Part model, mm, in its own coordinate system. A direction names the side the tool comes from. Round coordinates to 2 decimals unless told otherwise and drop trailing zeros. Write each question's results on one line, items separated by ' | '. Start each with the question number.
1. Drop flat-ended pins along their axis: pin 1 Ø3 at (x, z) = (-3, 5.5) entering from +Y; pin 2 Ø1 at (x, y) = (6.5, 12.5) entering from +Z; pin 3 Ø0.6 at (x, z) = (1, -5.5) entering from +Y. Give the stop position or say it passes through.
2. Which spindle directions (+Z, -Z, +X, -X, +Y, -Y) get a long thin tool onto all of the face, cutting with end or side? Do faces 4 (the face through (0, 4, -3)), 5 (the face through (0.1, 3.5, 0)), 6 (the face through (8.699, 0.285, 3.118)). Say none if no direction does.
3. Two-plate mould, pull along Z, no slides. Class faces 1 (the face through (0, 3, -2)), 2 (the face through (0.126, 4.285, -6.214)), 3 (the face through (0, 0, 4)): +Z half, -Z half, draft (parallel to the pull), parting line (faces both ways), or undercut.
4. Probe L1, parallel to Z at x = -4.75, y = 1; L2, parallel to Y at x = -6, z = -2.5; L3, parallel to Y at x = 5, z = -0.75. List the from-to ranges inside material, lowest first. Write a range as [from, to].
```python
from build123d import *

# Parameters (mm, degrees)
F1_DEPTH = 15
F4_DEPTH = 19
F5_R     = 1


with BuildPart() as f1:
    # F0 (on Front) → F1 (new body)
    with BuildSketch(Plane.XZ):
        Polygon((-9, 12.5), (-9, 0), (-9, -6.5152065011), (8.9999935767, -6.5152065011), (8.9999935767, 12.4847934989), align=None)
    extrude(amount=-F1_DEPTH)

    # F3 (on offset) → F4 (cut)
    with BuildSketch(Plane.YZ.offset(8.9999935767)):
        Polygon((3, -6.568428129), (3, -6.9065713324), (4, -6.9065713324), (4, 0), (3, 0), (3, -4.7258920968), (3.2896485645, -5.2308174782), (3.2896485645, -6.3381111249), align=None)
        with BuildLine():
            add(Edge.make_bspline(
                [(4, -6.9065713324), (7.8309681267, -7.469817996), (4.7241249122, 9.7180437297), (15.3055908158, 9.7582889721)],
                knots=[0, 0, 0, 0, 20.1378735884, 20.1378735884, 20.1378735884, 20.1378735884], degree=3))
            Line((4, -6.9065713324), (4, -7.8707002103))
            Line((4, -7.8707002103), (15.5558949336, -7.8707002103))
            Line((15.5558949336, -7.8707002103), (15.5558949336, -0.2191853659))
            Line((15.5558949336, -0.2191853659), (15.5479665846, 0.0968497843))
            Line((15.5479665846, 0.0968497843), (15.3055908158, 9.7582889721))
        make_face()
    extrude(amount=-F4_DEPTH, mode=Mode.SUBTRACT)

    # F5
    f5_edges = [f1.edges().sort_by_distance(p)[0] for p in [
        (-9, 0, 2.992397),
        (-3e-06, 0, -6.515207),
        (8.999994, 0, 2.984793),
        (-3e-06, 4, -6.515207),
    ]]
    fillet(f5_edges, radius=F5_R)


solid = f1.part
```
Solution:
1) pin 1: y = 9.57 | pin 2: z = 12.49 | pin 3: y = 5.7
2) face 4: -Z, +X, -X | face 5: +X, -X | face 6: +Z, -Z, +X, -Y
3) face 1: undercut | face 2: -Z half | face 3: draft
4) L1: [-6.52, 12.5] | L2: [0, 3], [4, 6.35] | L3: [0, 3], [4, 6.7]
